from build123d import *

# Parameters (mm, degrees)
F0_R     = 6.46875
F0_R_2   = 2.5
F1_DEPTH = 5.67817
F2_SIZE  = 2.38125
F3_W     = 10.46875
F3_H     = 12.9375
F4_DEPTH = 1.70942


with BuildPart() as f1:
    # F0 (on Top) → F1 (new body)
    with BuildSketch(Plane.XY):
        Circle(F0_R)
        Circle(F0_R_2, mode=Mode.SUBTRACT)
    extrude(amount=F1_DEPTH)

    # F2
    f2_edges = [f1.edges().sort_by_distance(p)[0] for p in [
        (-6.46875, 0, 0),
    ]]
    chamfer(f2_edges, length=F2_SIZE)

    # F3 (on face) → F4 (cut)
    with BuildSketch(Plane.XY.offset(5.67817)):
        with Locations((-1.234375, 0)):
            Rectangle(F3_W, F3_H)
    extrude(amount=-F4_DEPTH, mode=Mode.SUBTRACT)


solid = f1.part
Input: part model. Units: mm. Frame: model coordinates. A direction names the side the tool comes from. Coordinates: 2 decimals unless noted, no trailing zeros. Order: outer loops, then holes, each group sorted by start corner. A loop starts at its lowest first (then second) coordinate and runs counter-clockwise, first axis right, second up. Notation, with made-up numbers: M -38.75,27.25 L -12.75,27.25 A33 cw -12.75,59.25 Z; hole C 16,24 d7. An arc over 180 degrees is marked long. Answer in a Markdown table with one row per item.
(1) Access query for faces 5 (the flat face through (-2.5, -1.3, 3.969)), 6 (the flat face through (-2, -2, 0)). Directions: +Z, -Z, +X, -X, +Y, -Y. A direction counts if a zero-diameter tool reaches every point of the face in a straight line with its end or side. Return the directions, or none.
Numbers:
| item | result |
|---|---|
| face 5 | +Z, -X, +Y, -Y |
| face 6 | -Z, +X, -X, +Y, -Y |
(2) Section query A-A, the plane y = 0. Output: boundary loops of the cut face in (x, z).
Numbers:
| item | result |
|---|---|
| outline | M -6.47,2.38 L -4.09,0 L -2.5,0 L -2.5,3.97 L -6.47,3.97 Z; M 2.5,0 L 4.09,0 L 6.47,2.38 L 6.47,5.68 L 4,5.68 L 4,3.97 L 2.5,3.97 Z |
(3) Section query B-B, the plane x = 0. Output: boundary loops of the cut face in (y, z).
Numbers:
| item | result |
|---|---|
| outline | M -6.47,2.38 L -4.09,0 L -2.5,0 L -2.5,3.97 L -6.47,3.97 Z; M 2.5,0 L 4.09,0 L 6.47,2.38 L 6.47,3.97 L 2.5,3.97 Z |
(4) Section query D-D, the plane z = 2.85. Output: boundary loops of the cut face in (x, y), plus the area to 3 significant figures.
Numbers:
| item | result |
|---|---|
| outline | C 0,0 d12.94; hole C 0,0 d5 |
| area | 112 mm^2 |
(5) Material intervals for line 1 (Y direction, x = 0, z = 2.65); line 2 (Y direction, x = 0, z = 1.2), sorted ascending. Write a range as [from, to].
Numbers:
| item | result |
|---|---|
| line 1 | y = [-6.47, -2.5], [2.5, 6.47] |
| line 2 | y = [-5.29, -2.5], [2.5, 5.29] |
(6) Section query C-C, the plane z = 5.1. Output: boundary loops of the cut face in (x, y), plus the area to 3 significant figures.
Numbers:
| item | result |
|---|---|
| outline | M 4,-5.08 A6.47 ccw 4,5.08 Z |
| area | 17.5 mm^2 |
(7) Draft query along X for faces 1 (the flat face through (4, 0, 5)), 2 (the cylindrical face through (-0.54, -2.44, 1.96)), 3 (the flat face through (5, 0, 5.678)), 4 (the conical face through (-0.911, -4.103, 0.116)). Return one class per face: pulls with the +X half, pulls with the -X half, needs draft (parallel to the pull), parting line crosses it, or undercut.
Numbers:
| item | result |
|---|---|
| face 1 | pulls with the -X half |
| face 2 | undercut |
| face 3 | needs draft |
| face 4 | parting line crosses it |
(8) Contact query for flat-ended pins moving along their axis: pin 1 Ø1.5 at (x, y) = (-3.5, 5) entering from -Z; pin 2 Ø3 at (x, y) = (-2.5, 0) entering from +Z; pin 3 Ø1 at (y, z) = (-1, 3.5) entering from +X; pin 4 Ø4.5 at (x, y) = (0, 0) entering from +Z. Output: stop coordinate, or through.
Numbers:
| item | result |
|---|---|
| pin 1 | stops at z = 1.27 |
| pin 2 | stops at z = 3.97 |
| pin 3 | stops at x = 6.45 |
| pin 4 | passes through |
